```python
from build123d import *

# Parameters (mm, degrees)
SKETCH1_W           = 76.2
SKETCH1_H           = 87.7
SKETCH1_R           = 4.7625
BOSS_EXTRUDE1_DEPTH = 12.7
SKETCH2_R           = 12.5
SKETCH2_R_2         = 1.5875
CUT_EXTRUDE1_DEPTH  = 12.7


with BuildPart() as part:
    # Sketch1 → Boss-Extrude1 (new body)
    with BuildSketch(Plane(origin=(0, 0, 0), x_dir=(1, 0, 0), z_dir=(0, 1, 0))):
        with Locations((20.6375, -31.15)):
            Rectangle(SKETCH1_W, SKETCH1_H)
        Circle(SKETCH1_R, mode=Mode.SUBTRACT)
        with Locations((41.275, 0)):
            Circle(SKETCH1_R, mode=Mode.SUBTRACT)
    extrude(amount=BOSS_EXTRUDE1_DEPTH)

    # Sketch2 → Cut-Extrude1 (cut)
    with BuildSketch(Plane(origin=(0, 12.7, 0), x_dir=(1, 0, 0), z_dir=(0, 1, 0))):
        with Locations((20.6375, -44.45)):
            Circle(SKETCH2_R)
        with Locations((36.1375, -28.95)):
            Circle(SKETCH2_R_2)
        with Locations((5.1375, -28.95)):
            Circle(SKETCH2_R_2)
        with Locations((36.1375, -59.95)):
            Circle(SKETCH2_R_2)
        with Locations((5.1375, -59.95)):
            Circle(SKETCH2_R_2)
    extrude(amount=-CUT_EXTRUDE1_DEPTH, mode=Mode.SUBTRACT)


solid = part.part
```
The model under review builds one solid part; all positions refer to its coordinate system, in mm. Round coordinates to 2 decimals unless told otherwise and drop trailing zeros. Loops run counter-clockwise (first coordinate to the right, second up) from the corner with the lowest first, then second, coordinate; pieces in that order, holes last. Notation, with made-up numbers: M -19.5,-20 L 5.5,-20 A12 cw 5.5,-15 Z; hole C 79.5,-1.75 d10. An arc over 180 degrees is marked long. Put each result on its own line as item: value.
Q1. To check wall thickness, follow L1, parallel to X at y = 8.75, z = 0; L2, parallel to X at y = 5.75, z = -0.5; L3, parallel to Z at x = 20.5, y = 5. State the ranges of each line that lie inside material, in increasing order.
Result set:
L1: x = -17.46 to -4.76, 4.76 to 36.51, 46.04 to 58.74
L2: x = -17.46 to -4.74, 4.74 to 36.54, 46.01 to 58.74
L3: z = -12.7 to 31.95, 56.95 to 75
Q2. Consider section C-C, the plane z = 44.45. Give the boundary of the cut face in (x, y).
Result set:
outline: M -17.46,0 L 8.14,0 L 8.14,12.7 L -17.46,12.7 Z; M 33.14,0 L 58.74,0 L 58.74,12.7 L 33.14,12.7 Z
Q3. Consider section B-B, the plane z = 0. Give the boundary of the cut face in (x, y).
Result set:
outline: M -17.46,0 L -4.76,0 L -4.76,12.7 L -17.46,12.7 Z; M 4.76,0 L 36.51,0 L 36.51,12.7 L 4.76,12.7 Z; M 46.04,0 L 58.74,0 L 58.74,12.7 L 46.04,12.7 Z
Q4. Consider section A-A, the plane x = 0. Give the boundary of the cut face in (y, z).
Result set:
outline: M 0,-12.7 L 12.7,-12.7 L 12.7,-4.76 L 0,-4.76 Z; M 0,4.76 L 12.7,4.76 L 12.7,75 L 0,75 Z
Q5. Mouldability with a two-part tool opening along Z and no side actions: class faces 1 (the flat face through (20, 6, -12.7)), 2 (the flat face through (20, 0, 31)), 3 (the cylindrical face through (35.8, 6.4, 61.5)), 4 (the flat face through (20, 6, 75)) as released by +Z, released by -Z, zero draft, split by the parting line, or undercut.
Result set:
face 1: released by -Z
face 2: zero draft
face 3: undercut
face 4: released by +Z
Q6. Consider section D-D, the plane y = 5.75. Count the separate pieces of the cut face and the enclosed holes in it, then the cut area to 3 significant figures.
Result set:
separate pieces: 1
enclosed holes: 7
area: 6,020 mm²
